Here's how the part is built. I have some questions about the finished solid (model axes, mm). A direction names the side the tool comes from. Coordinates: 2 decimals unless noted, no trailing zeros. Write each loop counter-clockwise with the first axis right and the second up, starting at its lowest first coordinate (ties: lowest second). Pieces come first, ordered by that corner, then holes. Notation, with made-up numbers: (36, -18.75) -> (92, -18.75) arc R12 ccw to (92, -13.75) -> close; hole circle Ø1 at (41.5, 25). An arc over 180 degrees is marked (long way). Use CSV: the item, a comma, the result in double quotes. Start each with the question number.
```python
from build123d import *

# Parameters (mm, degrees)
BOSS_EXTRUDE1_DEPTH      = 64
BOSS_EXTRUDE1_DEPTH_BACK = 64
SKETCH1_R                = 63.5
CHAMFER1_SIZE            = 5
BOSS_EXTRUDE2_DEPTH      = 67.3
BOSS_EXTRUDE2_DEPTH_BACK = 66.5
SKETCH9_R                = 59
CHAMFER2_SIZE            = 5


with BuildPart() as part:
    # Sketch1 → Boss-Extrude1 (new, two sides: drawn at the far end of the back side and taken through both)
    with BuildSketch(Plane.XY.offset(-BOSS_EXTRUDE1_DEPTH_BACK)):
        Circle(SKETCH1_R)
    extrude(amount=BOSS_EXTRUDE1_DEPTH + BOSS_EXTRUDE1_DEPTH_BACK)

    # Chamfer1
    chamfer1_edges = [part.edges().sort_by_distance(p)[0] for p in [
        (-63.5, 0, 64),
    ]]
    chamfer(chamfer1_edges, length=CHAMFER1_SIZE)

    # Sketch6 for Loft1 → Loft1 section 0
    with BuildSketch(Plane.ZY):
        with BuildLine():
            Line((40.120383673, -54), (-42.379616327, -54))
            # circular arc as an exact rational Bezier (weights 1, cos(half-angle), 1)
            Bezier((-42.379616327, -54), (-75.725192624, 0), (-42.379616327, 54), weights=[1, 0.850849875, 1])
            Line((-42.379616327, 54), (40.120383673, 54))
            Bezier((40.120383673, 54), (79.472033784, 0), (40.120383673, -54), weights=[1, 0.80817386, 1])
        make_face()
    # Sketch7 for Loft1 → Loft1 section 1
    with BuildSketch(Plane(origin=(330.2, 0, 59), x_dir=(0, 0, 1), z_dir=(-1, 0, 0))):
        with BuildLine():
            Line((-21.003548385, -49.884), (-99.052818608, -49.884))
            Bezier((-99.052818608, -49.884), (-128.286627078, 0), (-99.052818608, 49.884), weights=[1, 0.862762376, 1])
            Line((-99.052818608, 49.884), (-21.003548385, 49.884))
            Bezier((-21.003548385, 49.884), (13.568719727, 0), (-21.003548385, -49.884), weights=[1, 0.821905309, 1])
        make_face()
    loft()

    # Sketch9 → Boss-Extrude2 (add, two sides: drawn at the far end of the back side and taken through both)
    with BuildSketch(Plane.XY.offset(-BOSS_EXTRUDE2_DEPTH_BACK)):
        with Locations((330.2, 0)):
            Circle(SKETCH9_R)
    extrude(amount=BOSS_EXTRUDE2_DEPTH + BOSS_EXTRUDE2_DEPTH_BACK)

    # Chamfer2
    chamfer2_edges = [part.edges().sort_by_distance(p)[0] for p in [
        (271.2, 0, -66.5),
    ]]
    chamfer(chamfer2_edges, length=CHAMFER2_SIZE)


solid = part.part
```
Item 1: I want a section at A-A on x = 0. Please give me the cut outline in (y, z), then the cut area to 3 significant figures.
Item 2: If I drill on line 1 along Z through (x, y) = (25.5, -21); line 2 along X through (y, z) = (-42, -58); line 3 along Y through (x, z) = (56.5, 0), over which ranges is the centre line in solid material (lowest first)?
Item 3: Thinking about a two-plate mould opening in X: for faces 1 (the conical face through (-7.65, 58.24, 63.76)), 2 (the cylindrical face through (-63.44, 2.79, -3.36)), 3 (the flat face through (329, 1, -66.5)), which applies, +X half, -X half, draft (parallel to the pull), parting line (faces both ways), or undercut?
Item 4: Which directions (+Z, -Z, +X, -X, +Y, -Y) give clear straight access to the entire face, cutting with the end or side of a thin tool? Please do faces 4 (the flat face through (-1, 1, -64)), 5 (the flat face through (329, 1, 67.3)), 6 (the flat face through (-1, 1, 64)).
Item 5: I'm going to push flat-ended pins straight in: pin 1 (3 mm diameter, centred on y = 27, z = 42.5, fed in from +X); pin 2 (3 mm diameter, centred on y = 49.5, z = -24, fed in from +X); pin 3 (10 mm diameter, centred on y = -27, z = 34, fed in from +X). Where does each tip first touch, or does it pass through?
Geometry says:
1,outline,"(-63.5, -64) -> (63.5, -64) -> (63.5, 59) -> (58.5, 64) -> (-58.5, 64) -> (-63.5, 59) -> close"
1,area,"16,200 mm2"
2,line 1,"-64 to 64"
2,line 2,"-47.63 to 47.63, 288.76 to 371.64"
2,line 3,"-53.3 to 53.3"
3,face 1,"undercut"
3,face 2,"undercut"
3,face 3,"draft"
4,face 4,"-Z, -X, +Y, -Y"
4,face 5,"+Z, +X, -X, +Y, -Y"
4,face 6,"+Z, -X, +Y, -Y"
5,pin 1,"x = 383.4"
5,pin 2,"x = 364.51"
5,pin 3,"x = 384.94"
